Verification items for this drawing (mm, ordinates from the low corner). Round coordinates to 2 decimals unless told otherwise and drop trailing zeros. Write each loop counter-clockwise with the first axis right and the second up, starting at its lowest first coordinate (ties: lowest second). Pieces come first, ordered by that corner, then holes.
Item 1: Draft check along X on the marked faces 1, 2, 3 and 4. Enter one of: pulls with the +X half, pulls with the -X half, needs draft (parallel to the pull), parting line crosses it, or undercut.
Item 2: Cross-section at D-D (x = 45). Enter the section's corners in (y, z).
Item 3: Scan lines: probe 1 along Y at (x, z) = (40, 1); probe 2 along Y at (x, z) = (60, 2.55); probe 3 along Y at (x, z) = (25, 0.95). Record each from-to range of solid material in increasing order.
Item 4: Cross-section at C-C (y = 70). Enter the section's corners in (x, z).
Item 5: Depth check by flat-ended pin: P1, Ø2.5, axis at x = 10, y = 70, coming from the -Z side; P2, Ø13, axis at x = 25, y = 30, coming from the +Z side. Enter the tip coordinate at first touch or a pass-through.
Item 6: Cross-section at A-A (x = 25). Enter the section's corners in (y, z), then the cut area to 3 significant figures.
Item 7: Cross-section at B-B (y = 50). Enter the section's corners in (x, z), then the cut area to 3 significant figures.
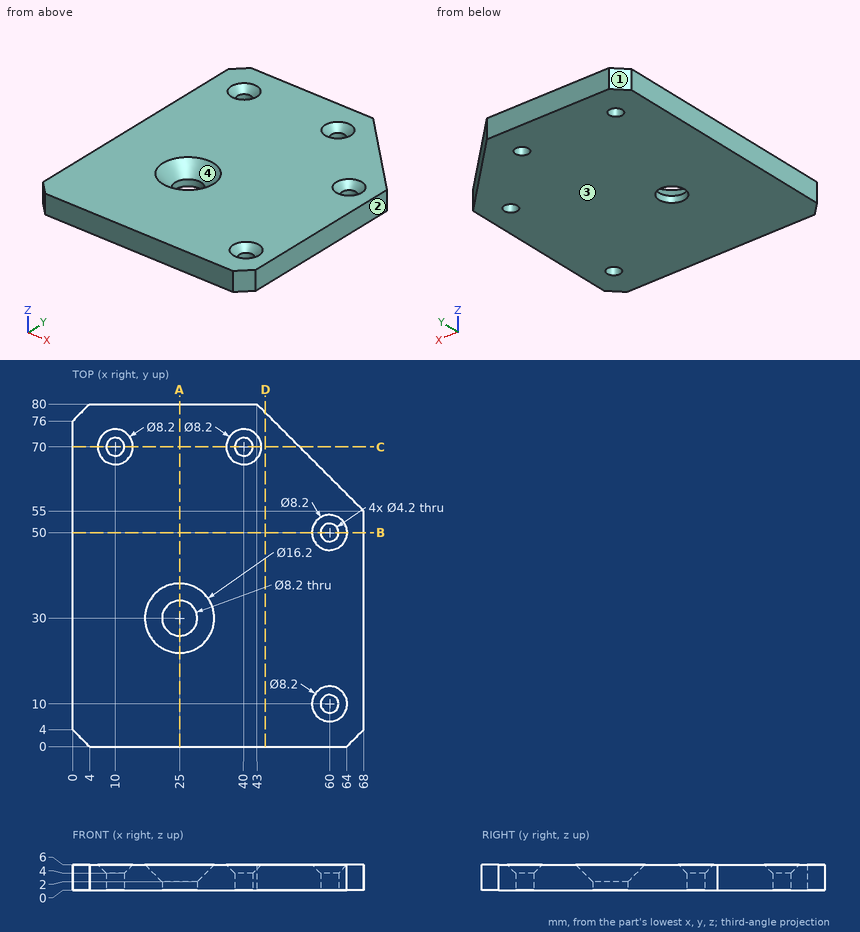
Resolved:
1. face 1: pulls with the -X half
1. face 2: pulls with the +X half
1. face 3: needs draft
1. face 4: undercut
2. outline: (0, 0) - (78, 0) - (78, 6) - (0, 6) - close
3. probe 1: y = 0 to 67.9, 72.1 to 80
3. probe 2: y = 0 to 7.9, 12.1 to 47.9, 52.1 to 63
3. probe 3: y = 0 to 25.9, 34.1 to 80
4. outline: (0, 0) - (7.9, 0) - (7.9, 4) - (5.9, 6) - (0, 6) - close; (12.1, 0) - (37.9, 0) - (37.9, 4) - (35.9, 6) - (14.1, 6) - (12.1, 4) - close; (42.1, 0) - (53, 0) - (53, 6) - (44.1, 6) - (42.1, 4) - close
5. P1: passes through
5. P2: stops at z = 4.4
6. outline: (0, 0) - (25.9, 0) - (25.9, 2) - (21.9, 6) - (0, 6) - close; (34.1, 0) - (80, 0) - (80, 6) - (38.1, 6) - (34.1, 2) - close
6. area: 415 mm2
7. outline: (0, 0) - (57.9, 0) - (57.9, 4) - (55.9, 6) - (0, 6) - close; (62.1, 0) - (68, 0) - (68, 6) - (64.1, 6) - (62.1, 4) - close
7. area: 379 mm2
